```python
from build123d import *

# Parameters (mm, degrees)
BOSS_EXTRUDE1_DEPTH                = 12.9032
BOSS_EXTRUDE2_DEPTH                = 0.508
CUT_EXTRUDE1_DEPTH                 = 12.9032
BOSS_EXTRUDE3_DEPTH                = 1.2954
CUT_EXTRUDE2_DEPTH                 = 0.508
BOSS_EXTRUDE4_DEPTH                = 0.3048
BOSS_EXTRUDE5_DEPTH                = 0.508
SKETCH8_W                          = 412.6484
SKETCH8_H                          = 0.508
CUT_EXTRUDE3_DEPTH                 = 0.3048
SKETCH9_W                          = 412.6484
SKETCH9_H                          = 1.8034
BOSS_EXTRUDE6_DEPTH                = 1.2954
SKETCH10_W                         = 412.6484
SKETCH10_H                         = 0.508
CUT_EXTRUDE4_DEPTH                 = 0.508
SKETCH11_W                         = 412.6484
SKETCH11_H                         = 1.2954
BOSS_EXTRUDE7_DEPTH                = 12.9032
SKETCH12_W                         = 5.8166
SKETCH12_H                         = 1.2954
BOSS_EXTRUDE8_DEPTH                = 2.1082
SKETCH13_W                         = 5.8166
SKETCH13_H                         = 1.2954
BOSS_EXTRUDE9_DEPTH                = 2.1082
HOLE1_D                            = 4.953
HOLE1_DEPTH                        = 1.2954
F_3_16_0_1875_DIAMETER_HOLE1_D     = 4.7625
F_3_16_0_1875_DIAMETER_HOLE1_DEPTH = 78.6892
FILLET1_R                          = 0.508
FILLET2_R                          = 1.8034
FILLET3_R                          = 1.904999999
CUT_EXTRUDE5_DEPTH                 = 435.13094631


with BuildPart() as part:
    # Sketch1 → Boss-Extrude1 (new body)
    with BuildSketch(Plane.XZ.offset(-290.0934)):
        Polygon((426.4406, 80.2386), (1.5494, 80.2386), (1.5494, 78.9432), (1.5494, 78.4352), (1.5494, 3.6576), (426.4406, 3.6576), (426.4406, 78.4352), (426.4406, 78.9432), align=None)
    extrude(amount=-BOSS_EXTRUDE1_DEPTH)

    # Sketch2 → Boss-Extrude2 (add)
    with BuildSketch(Plane(origin=(0, 302.9966, 0), x_dir=(-1, 0, 0), z_dir=(0, 1, 0))):
        Polygon((-1.5494, 3.6576), (-426.4406, 3.6576), (-426.4406, 78.4352), (-426.4406, 78.943205), (-426.4406, 80.2386), (-1.5494, 80.2386), (-1.5494, 78.943205), (-1.5494, 78.4352), align=None)
    extrude(amount=BOSS_EXTRUDE2_DEPTH)

    # Sketch3 → Cut-Extrude1 (cut)
    with BuildSketch(Plane.XZ.offset(-290.0934)):
        Polygon((1.5494, 3.6576), (426.4406, 3.6576), (426.4406, 78.4352), (426.4406, 78.9432), (1.5494, 78.9432), (1.5494, 78.4352), align=None)
    extrude(amount=-CUT_EXTRUDE1_DEPTH, mode=Mode.SUBTRACT)

    # Sketch4 → Boss-Extrude3 (add)
    with BuildSketch(Plane(origin=(0, 303.5046, 0), x_dir=(-1, 0, 0), z_dir=(0, 1, 0))):
        Polygon((-1.5494, 3.6576), (-426.4406, 3.6576), (-426.4406, 78.4352), (-426.4406, 80.2386), (-1.5494, 80.2386), (-1.5494, 78.4352), align=None)
    extrude(amount=BOSS_EXTRUDE3_DEPTH)

    # Sketch5 → Cut-Extrude2 (cut)
    with BuildSketch(Plane.XZ.offset(-302.9966)):
        Polygon((1.5494, 3.6576), (426.4406, 3.6576), (426.4406, 78.4352), (426.4406, 78.9432), (1.5494, 78.9432), (1.5494, 78.4352), align=None)
    extrude(amount=-CUT_EXTRUDE2_DEPTH, mode=Mode.SUBTRACT)

    # Sketch6 → Boss-Extrude4 (add)
    with BuildSketch(Plane(origin=(0, 0, 3.6576), x_dir=(-1, 0, 0), z_dir=(0, 0, -1))):
        Polygon((-420.3192, 302.9966), (-420.3192, 303.5046), (-420.3192, 304.8), (-7.6708, 304.8), (-7.6708, 303.5046), (-7.6708, 302.9966), align=None)
    extrude(amount=BOSS_EXTRUDE4_DEPTH)

    # Sketch7 → Boss-Extrude5 (add)
    with BuildSketch(Plane(origin=(0, 0, 3.3528), x_dir=(-1, 0, 0), z_dir=(0, 0, -1))):
        Polygon((-420.3192, 302.9966), (-420.3192, 303.5046), (-420.3192, 304.8), (-7.6708, 304.8), (-7.6708, 303.504605), (-7.6708, 302.9966), align=None)
    extrude(amount=BOSS_EXTRUDE5_DEPTH)

    # Sketch8 → Cut-Extrude3 (cut)
    with BuildSketch(Plane.XY.offset(3.6576)):
        with Locations((213.995, 303.2506)):
            Rectangle(SKETCH8_W, SKETCH8_H)
    extrude(amount=-CUT_EXTRUDE3_DEPTH, mode=Mode.SUBTRACT)

    # Sketch9 → Boss-Extrude6 (add)
    with BuildSketch(Plane(origin=(0, 0, 2.8448), x_dir=(-1, 0, 0), z_dir=(0, 0, -1))):
        with Locations((-213.995, 303.8983)):
            Rectangle(SKETCH9_W, SKETCH9_H)
    extrude(amount=BOSS_EXTRUDE6_DEPTH)

    # Sketch10 → Cut-Extrude4 (cut)
    with BuildSketch(Plane.XY.offset(3.3528)):
        with Locations((213.995, 303.2506)):
            Rectangle(SKETCH10_W, SKETCH10_H)
    extrude(amount=-CUT_EXTRUDE4_DEPTH, mode=Mode.SUBTRACT)

    # Sketch11 → Boss-Extrude7 (add)
    with BuildSketch(Plane.XZ.offset(-302.9966)):
        with Locations((213.995, 2.1971)):
            Rectangle(SKETCH11_W, SKETCH11_H)
    extrude(amount=BOSS_EXTRUDE7_DEPTH)

    # Sketch12 → Boss-Extrude8 (add)
    with BuildSketch(Plane(origin=(0, 0, 3.6576), x_dir=(-1, 0, 0), z_dir=(0, 0, -1))):
        with Locations((-4.4577, 304.1523)):
            Rectangle(SKETCH12_W, SKETCH12_H)
    extrude(amount=BOSS_EXTRUDE8_DEPTH)

    # Sketch13 → Boss-Extrude9 (add)
    with BuildSketch(Plane(origin=(0, 0, 3.6576), x_dir=(-1, 0, 0), z_dir=(0, 0, -1))):
        with Locations((-423.5323, 304.1523)):
            Rectangle(SKETCH13_W, SKETCH13_H)
    extrude(amount=BOSS_EXTRUDE9_DEPTH)

    # Hole1
    with Locations(Plane(origin=(0, 0, 1.5494), x_dir=(-1, 0, 0), z_dir=(0, 0, -1))):
        with Locations((-213.995, 295.9989), (-393.1666, 295.9989), (-34.8234, 295.9989)):
            Hole(HOLE1_D / 2, depth=HOLE1_DEPTH)

    # 3/16 (0.1875) Diameter Hole1
    with Locations(Plane.XY.offset(80.2386)):
        with Locations((34.8234, 295.68775), (213.995, 295.68775), (393.1666, 295.68775)):
            Hole(F_3_16_0_1875_DIAMETER_HOLE1_D / 2, depth=F_3_16_0_1875_DIAMETER_HOLE1_DEPTH)

    # Fillet1
    fillet1_edges = [part.edges().sort_by_distance(p)[0] for p in [
        (213.995, 303.5046, 2.8448),
        (1.5494, 304.1523, 1.5494),
        (426.4406, 304.1523, 1.5494),
        (213.995, 303.5046, 78.9432),
    ]]
    fillet(fillet1_edges, radius=FILLET1_R)

    # Fillet2
    fillet2_edges = [part.edges().sort_by_distance(p)[0] for p in [
        (213.995, 304.8, 1.5494),
        (213.995, 304.8, 80.2386),
    ]]
    fillet(fillet2_edges, radius=FILLET2_R)

    # Fillet3
    fillet3_edges = [part.edges().sort_by_distance(p)[0] for p in [
        (420.3192, 290.0934, 2.1971),
        (7.6708, 290.0934, 2.1971),
        (426.4406, 290.0934, 79.5909),
        (1.5494, 290.0934, 79.5909),
    ]]
    fillet(fillet3_edges, radius=FILLET3_R)

    # Sketch18 → Cut-Extrude5 (cut, through all)
    with BuildSketch(Plane.XZ.offset(-303.5046)):
        with BuildLine():
            Line((357.505, 50.3682), (292.735, 50.3682))
            ThreePointArc((292.735, 50.3682), (290.938948776, 49.624251224), (290.195, 47.8282))
            Line((290.195, 47.8282), (290.195, 33.8582))
            ThreePointArc((290.195, 33.8582), (290.938948776, 32.062148776), (292.735, 31.3182))
            Line((292.735, 31.3182), (357.505, 31.3182))
            ThreePointArc((357.505, 31.3182), (359.301051224, 32.062148776), (360.045, 33.8582))
            Line((360.045, 33.8582), (360.045, 47.8282))
            ThreePointArc((360.045, 47.8282), (359.301051224, 49.624251224), (357.505, 50.3682))
        make_face()
        with BuildLine():
            Line((137.795, 47.8282), (137.795, 33.8582))
            ThreePointArc((137.795, 33.8582), (137.051051224, 32.062148776), (135.255, 31.3182))
            Line((135.255, 31.3182), (70.485, 31.3182))
            ThreePointArc((70.485, 31.3182), (68.688948776, 32.062148776), (67.945, 33.8582))
            Line((67.945, 33.8582), (67.945, 47.8282))
            ThreePointArc((67.945, 47.8282), (68.688948776, 49.624251224), (70.485, 50.3682))
            Line((70.485, 50.3682), (135.255, 50.3682))
            ThreePointArc((135.255, 50.3682), (137.051051224, 49.624251224), (137.795, 47.8282))
        make_face()
    extrude(amount=-CUT_EXTRUDE5_DEPTH, mode=Mode.SUBTRACT)


solid = part.part
```
Check sheet for the modelled part. Datum: model origin and axes. Units: mm. A direction names the side the tool comes from. Round coordinates to 2 decimals unless told otherwise and drop trailing zeros. Loops run counter-clockwise (first coordinate to the right, second up) from the corner with the lowest first, then second, coordinate; pieces in that order, holes last. Notation, with made-up numbers: (61.5, 87.25) - (80.5, 87.25) arc R23 cw to (80.5, 109.25) - close; hole circle Ø9 at (84, 16). An arc over 180 degrees is marked (long way). Write item = value, one per line. Start each with the question number.
Q1. Depth check by flat-ended pin: P1, Ø1, axis at x = 311, y = 304, coming from the -Z side; P2, Ø0.6, axis at y = 297, z = 2.5, coming from the -X side; P3, Ø0.6, axis at x = 88, y = 304, coming from the +Z side. Enter the tip coordinate at first touch or a pass-through.
Q2. Access from +Z, -Z, +X, -X, +Y, -Y to the whole of each face (thin tool, end or side, straight path). Record for faces 1 (the face through (426.441, 304, 50)), 2 (the face through (211, 297, 2.845)).
Q3. Section check C-C (x = 373). Record the boundary of the cut face in (y, z), plus the area to 3 significant figures.
Q4. Thickness scan on L1, parallel to Z at x = 232.5, y = 292; L2, parallel to Y at x = 51.5, z = 40; L3, parallel to Z at x = 36, y = 303.25. Record the ranges inside material, lowest first.
Q5. Release check for a two-part mould opening along Z. For faces 3 (the face through (211, 297, 1.549)), 4 (the face through (217, 303.505, 41)), 5 (the face through (217, 304.8, 41)), 6 (the face through (217, 296, 80.239)) record: pulls with the +Z half, pulls with the -Z half, needs draft (parallel to the pull), parting line crosses it, or undercut.
Q6. Section check A-A (x = 131.5). Record the boundary of the cut face in (y, z), plus the area to 3 significant figures.
Q7. Section check B-B (z = 39.5). Record the boundary of the cut face in (x, y) (3 decimals).
Derived:
q1.P1 = 1.62
q1.P2 = 7.67
q1.P3 = 80.1
q2.face_1 = +Z, -Z, +X, +Y, -Y
q2.face_2 = +X, -X, -Y
q3.outline = (290.09, 1.55) - (303, 1.55) arc R1.8 ccw to (304.8, 3.35) - (304.8, 78.44) arc R1.8 ccw to (303, 80.24) - (290.09, 80.24) - (290.09, 78.94) - (303, 78.94) arc R0.51 cw to (303.5, 78.44) - (303.5, 3.35) arc R0.51 cw to (303, 2.84) - (290.09, 2.84) - close
q3.area = 135 mm^2
q4.L1 = 1.55 to 2.84, 78.94 to 80.24
q4.L2 = 303.5 to 304.8
q4.L3 = 1.57 to 2.91, 78.88 to 80.22
q5.face_3 = pulls with the -Z half
q5.face_4 = undercut
q5.face_5 = needs draft
q5.face_6 = pulls with the +Z half
q6.outline = (290.09, 1.55) - (303, 1.55) arc R1.8 ccw to (304.8, 3.35) - (304.8, 31.32) - (303.5, 31.32) - (303.5, 3.35) arc R0.51 cw to (303, 2.84) - (290.09, 2.84) - close; (290.09, 78.94) - (303, 78.94) arc R0.51 cw to (303.5, 78.44) - (303.5, 50.37) - (304.8, 50.37) - (304.8, 78.44) arc R1.8 ccw to (303, 80.24) - (290.09, 80.24) - close
q6.area = 111 mm^2
q7.outline = (1.549, 303.505) - (67.945, 303.505) - (67.945, 304.8) - (1.549, 304.8) - close; (137.795, 303.505) - (290.195, 303.505) - (290.195, 304.8) - (137.795, 304.8) - close; (360.045, 303.505) - (426.441, 303.505) - (426.441, 304.8) - (360.045, 304.8) - close
